Answer from the drawing. Dimensions are ordinates in mm from the lowest x, y and z of the part. Round coordinates to 2 decimals unless told otherwise and drop trailing zeros. Write each loop counter-clockwise with the first axis right and the second up, starting at its lowest first coordinate (ties: lowest second). Pieces come first, ordered by that corner, then holes. Notation, with made-up numbers: (-2, -26) - (23, -26) arc R27 cw to (23, -1) - close; hole circle Ø1 at (60, 67.5). An arc over 180 degrees is marked (long way). Use a Markdown table: item, result. Add a question column.
1) Find the intervals of material crossed by probe 1 along Y at (x, z) = (78, 0.75) (1 decimal); probe 2 along X at (y, z) = (38.5, 2.5) (1 decimal); probe 3 along X at (y, z) = (25, 5.25) (1 decimal), in increasing order. Write a range as from..to.
2) Determine the mould class of the marked faces 1 and 2 for opening direction X: +X half, -X half, draft (parallel to the pull), parting line (faces both ways), or undercut.
3) A cutting plane is placed at A-A (z = 3). Give the vertices of the cut face in (x, y) (1 decimal).
4) A cutting plane is placed at B-B (z = 9.25). Give the vertices of the cut face in (x, y) (1 decimal).
5) Each of these flat-tipped pins is pushed along its axis until it touches: P1, Ø5, axis at y = 10.5, z = 7, coming from the +X side (1 decimal); P2, Ø10, axis at x = 77.5, y = 49.5, coming from the -Z side (1 decimal); P3, Ø2, axis at y = 28.5, z = 6.5, coming from the -X side. Where does it stop, or does it pass through?
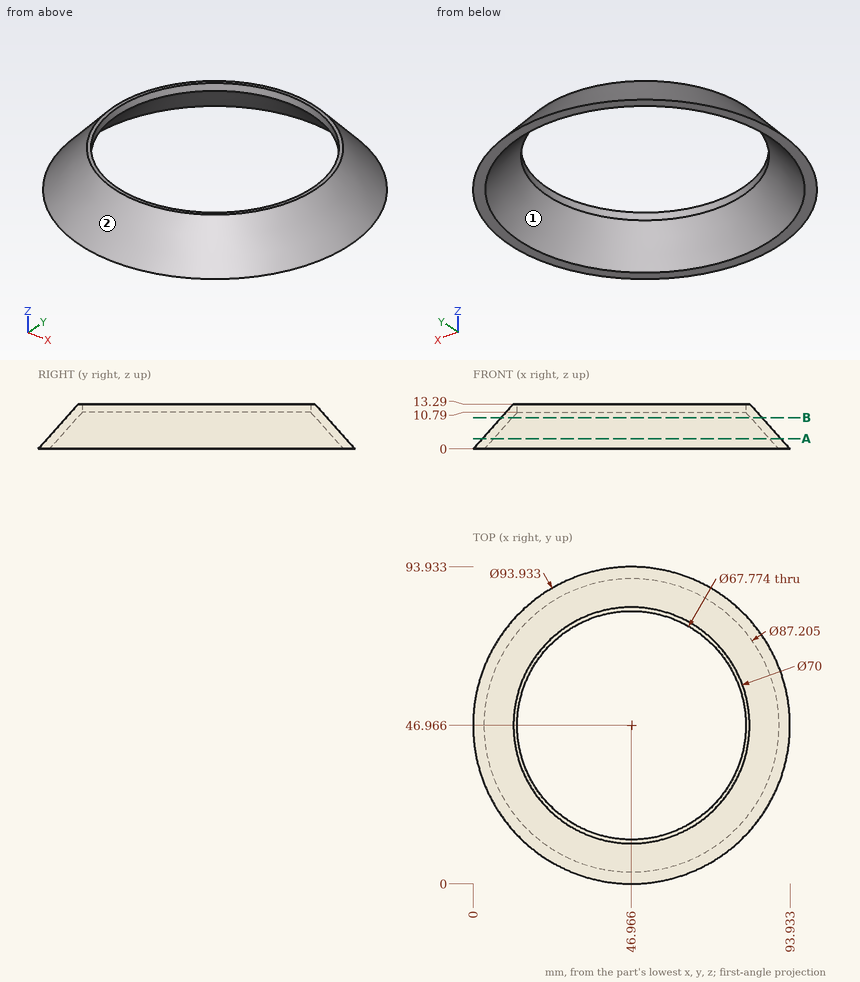
Entries:
| question | item | result |
|---|---|---|
| 1 | probe 1 | y = 12.6..17.3, 76.6..81.3 |
| 1 | probe 2 | x = 3.1..6.5, 87.4..90.9 |
| 1 | probe 3 | x = 10.9..14.9, 79..83 |
| 2 | face 1 | undercut |
| 2 | face 2 | parting line |
| 3 | outline | circle Ø88.5 at (47, 47); hole circle Ø81.8 at (47, 47) |
| 4 | outline | circle Ø77.3 at (47, 47); hole circle Ø70.5 at (47, 47) |
| 5 | P1 | stops at x = 71.1 |
| 5 | P2 | stops at z = 8.8 |
| 5 | P3 | stops at x = 9.12 |
